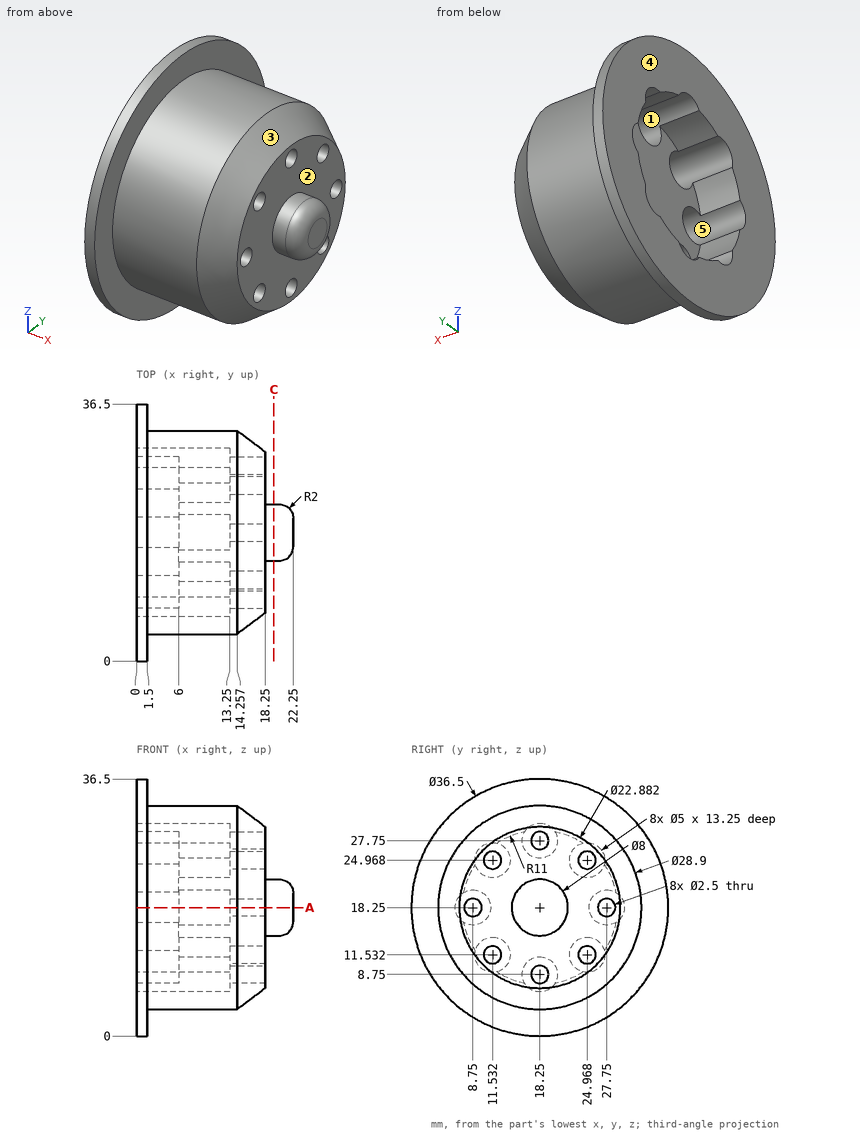
Study the drawing (mm; zero at the part's minimum x, y, z) and answer. A direction names the side the tool comes from. Round coordinates to 2 decimals unless told otherwise and drop trailing zeros. Loops run counter-clockwise (first coordinate to the right, second up) from the corner with the lowest first, then second, coordinate; pieces in that order, holes last. Notation, with made-up numbers: (29.25, -40) -> (59.25, -40) arc R6 ccw to (59.25, -33) -> close; hole circle Ø7 at (79.25, 10). An arc over 180 degrees is marked (long way). Use one line per item in the form item = value.
1. The part is cut by section C-C on x = 19.5. Determine the outline of the cut face in (y, z).
Answer key:
outline = circle Ø8 at (18.25, 18.25)
2. Flat-ended cylindrical pins translate along their axes: pin 1 Ø4 at (x, z) = (10, 29.5) entering from -Y; pin 2 Ø4 at (y, z) = (21.5, 26.5) entering from +X; pin 3 Ø4 at (x, y) = (13.5, 11.5) entering from -Z; pin 4 Ø17.5 at (y, z) = (17.5, 22.5) entering from -X. Find the tip coordinate at first contact, or state that the pin passes through.
Answer key:
pin_1 = 7.15
pin_2 = 18.25
pin_3 = 4.6
pin_4 = 0
3. Find the intervals of material crossed by probe 1 along Z at (x, y) = (8.25, 16) (1 decimal); probe 2 along Z at (x, y) = (14.5, 25.5) (1 decimal); probe 3 along X at (y, z) = (34, 19), in increasing order. Write a range as [from, to].
Answer key:
probe_1 = [4, 7.7], [9.8, 26.7], [28.8, 32.5]
probe_2 = [6, 10.4], [12.7, 23.8], [26.1, 30.5]
probe_3 = [0, 1.5]
4. For a pull along Y with two mould halves and no side action, classify the marked faces 3, 4 and 5 as released by +Y, released by -Y, zero draft, split by the parting line, or undercut.
Answer key:
face_3 = split by the parting line
face_4 = zero draft
face_5 = undercut
5. A tool of negligible diameter and unlimited length cuts with its end or side. For the marked faces 1 and 2, from which of +Z, -Z, +X, -X, +Y, -Y can it reach the whole face along a straight path? Write none if from no direction.
Answer key:
face_1 = -X
face_2 = +X
6. The part is cut by section A-A on z = 18.25. Give the number of separate pieces and of enclosed holes in the cut face.
Answer key:
separate_pieces = 3
enclosed_holes = 0
